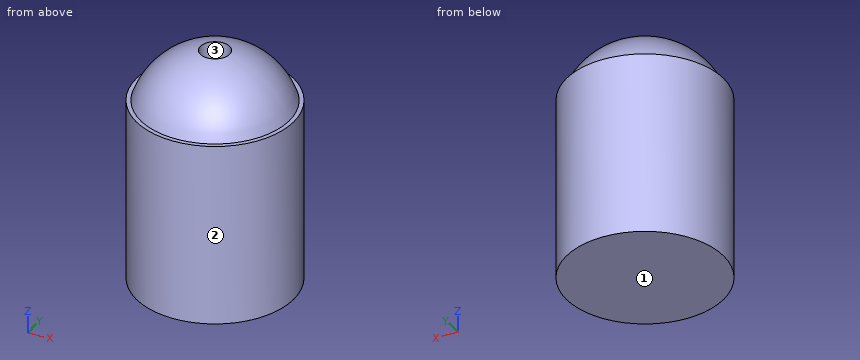
from build123d import *

# Parameters (mm, degrees)
F0_R     = 15
F1_DEPTH = 35
F5_R     = 2.792343
F6_DEPTH = 20


with BuildPart() as f1:
    # F0 (on Top) → F1 (new body)
    with BuildSketch(Plane.XY):
        Circle(F0_R)
    extrude(amount=F1_DEPTH)

    # F2 (on Front) → F3 (revolve)
    with BuildSketch(Plane.XZ):
        with BuildLine():
            Line((0, 29.952514), (0, 45.102068))
            ThreePointArc((0, 45.102068), (-10.659346, 40.655662), (-14.999254, 29.952514))
            Line((-14.999254, 29.952514), (0, 29.952514))
        make_face()
    revolve(axis=Axis((0, 0, 30.102068), (0, 0, -1)))

    # F5 (on offset) → F6 (cut)
    with BuildSketch(Plane.XY.offset(52.5)):
        Circle(F5_R)
    extrude(amount=-F6_DEPTH, mode=Mode.SUBTRACT)


solid = f1.part
Work out the finished part from the listing and answer in its coordinate system (mm). Face numbers are marked on the shaded views. Round coordinates to 2 decimals unless told otherwise and drop trailing zeros. Loops run counter-clockwise (first coordinate to the right, second up) from the corner with the lowest first, then second, coordinate; pieces in that order, holes last. Notation, with made-up numbers: (89.25, -22.75) - (147.25, -22.75) arc R13 ccw to (147.25, -8.75) - close; hole circle Ø5 at (-39, 4.25). An arc over 180 degrees is marked (long way). Use one line per item in the form item = value. Start each with the question number.
(1) Consider line 1 (Y direction, x = 0, z = 42); line 2 (X direction, y = 0, z = 40.25); line 3 (Y direction, x = 0, z = 42.25). Determine where each line is inside the solid, lowest interval first.
(2) Determine the mould class of the marked faces 1, 2 and 3 for opening direction X: +X half, -X half, draft (parallel to the pull), parting line (faces both ways), or undercut.
(3) Flat-ended cylindrical pins translate along their axes: P1, Ø2, axis at x = -7.5, z = 7.5, coming from the -Y side; P2, Ø1.7, axis at x = -0.5, y = 1.5, coming from the +Z side; P3, Ø4, axis at y = 3.5, z = 35.5, coming from the +X side. Find the tip coordinate at first contact, or state that the pin passes through.
(4) Find section A-A on z = 22.5. Determine the outline of the cut face in (x, y), and give its area (3 significant figures).
Answer list:
q1.line_1 = -9.13 to -2.79, 2.79 to 9.13
q1.line_2 = -11.05 to -2.79, 2.79 to 11.05
q1.line_3 = -8.8 to -2.79, 2.79 to 8.8
q2.face_1 = draft
q2.face_2 = parting line
q2.face_3 = undercut
q3.P1 = -13.52
q3.P2 = 32.5
q3.P3 = 14.92
q4.outline = circle Ø30 at (0, 0)
q4.area = 707 mm^2
